The listing builds one solid part. Answer for the finished solid, in the listing's coordinates (mm). Face numbers are marked on the shaded views. A direction names the side the tool comes from. Coordinates: 2 decimals unless noted, no trailing zeros. Loops run counter-clockwise (first coordinate to the right, second up) from the corner with the lowest first, then second, coordinate; pieces in that order, holes last. Notation, with made-up numbers: (53, 79.5) - (82, 79.5) arc R15 ccw to (82, 99.5) - close; hole circle Ø3 at (41, 53.5). An arc over 180 degrees is marked (long way). Return JSON: item names as keys, results as strings. Group by question number.
1. Which of the six approach directions +Z, -Z, +X, -X, +Y, -Y give full straight-line access (tool end or side, diameter ignored) to the marked faces 1 and 2?
2. Section A-A (x = 0) is taken. Write down the section's boundary in (y, z).
3. Find the intervals of material crossed by line 1 along X through (y, z) = (29, 1); line 2 along Y through (x, z) = (65, 4.5); line 3 along Z through (x, y) = (-253.5, 48.5), in increasing order.
4. Section C-C (x = 407) is taken. Write down the section's boundary in (y, z).
5. Section B-B (z = 16.25) is taken. Write down the section's boundary in (x, y).
6. Each of these flat-tipped pins is pushed along its axis until it touches: P1, Ø12, axis at x = 45, z = 12, coming from the +Y side; P2, Ø1.6, axis at x = -244.5, z = 1, coming from the +Y side; P3, Ø6, axis at x = -341.5, y = 37, coming from the +Z side. Where does it stop, or does it pass through?
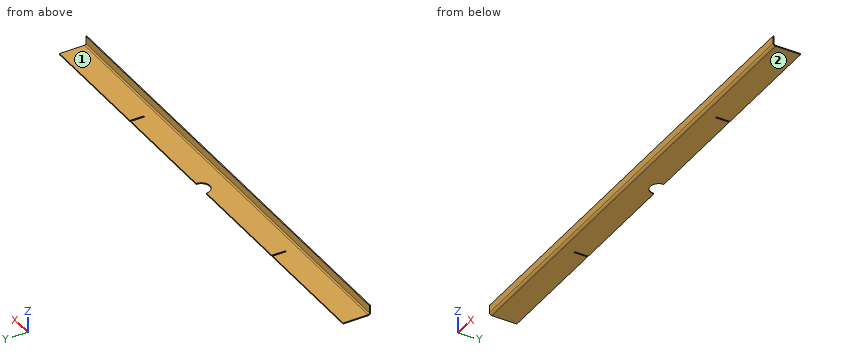
Autodesk Inventor part; units mm, degrees
ref_plane "YZ Plane" through (0, 0, 0) normal (1, 0, 0) x (0, 1, 0)
ref_plane "XZ Plane" through (0, 0, 0) normal (0, 1, 0) x (-1, 0, 0)
ref_plane "XY Plane" through (0, 0, 0) normal (0, 0, 1) x (1, 0, 0)
sketch "Sketch1" plane through (0, 0, 0) normal (0, 0, 1) x (1, 0, 0)
  line L0 (-490, 54) -> (490, 54)
  line L1 (490, 54) -> (490, 0)
  line L2 (490, 0) -> (-490, 0)
  line L3 (-490, 0) -> (-490, 54)
  point P0 (0, 0)
  point P1 (0, 0)
  dimension "d0" = 980
  dimension "d1" = 54
extrude "Plate1" add sketch "Sketch1" along normal blind 2
sketch "Sketch2" plane through (490, -2, 0) normal (0, 1, 0) x (-1, 0, 0)
  line L0 (980, 0) -> (0, 0)
  line L1 (0, 0) -> (0, 20)
  line L2 (0, 20) -> (980, 20)
  line L3 (980, 20) -> (980, 0)
edge flange "Flange1" height 20 angle 90 thickness 2 bend radius 2.75 thickness toward (0, 1, 0) relief round relief width 2 relief depth 1 edges at (0, 0, 2) wall of the first edge with corners at (-490, -2, 0) (490, -2, 0) (490, -2, 20) (-490, -2, 20)
bend "Bend1"
corner "Corner1"
sketch "Sketch5" plane through (0, 0, 0) normal (0, 0, -1) x (-1, 0, 0)
  line L0 (490, 54) -> (-490, 54)
  line L1 (490, -2) -> (-490, -2)
  circle A0 centre (0, 54) radius 17.5
  line L2 (243.4, 54) -> (246.6, 54)
  line L3 (246.6, 54) -> (246.6, 26)
  line L4 (246.6, 26) -> (243.4, 26)
  line L5 (243.4, 26) -> (243.4, 54)
  line L6 (-243.4, 54) -> (-246.6, 54)
  line L7 (-246.6, 54) -> (-246.6, 26)
  line L8 (-246.6, 26) -> (-243.4, 26)
  line L9 (-243.4, 26) -> (-243.4, 54)
  line L10 (0, 54) -> (0, -2) construction
  point P0 (0, 0)
  point P1 (-490, -2)
  point P2 (245, 26)
  point P3 (-245, 26)
  point P4 (246.6, 54)
  point P5 (-17.5, 54)
  point P6 (17.5, 54)
  point P7 (-246.6, 54)
  dimension "d45" = 35
  dimension "d48" = 3.2
  dimension "d49" = 490
  dimension "d51" = 28
  dimension "d52" = 28
extrude "Extrusion1" cut sketch "Sketch5" against normal through all contours L3 L4 L5 L0 | L9 L8 L7 L0 | A0 L0 picked at (-2.238, 47.1497)
sketch "Sketch9" plane through (0, 0, 2) normal (0, 0, 1) x (1, 0, 0)
  line L0 (485.6141, 29.596) -> (485.6141, 17.596) construction
  line L1 (485.6141, 17.596) -> (285.6141, 17.596) construction
  line L2 (285.6141, 17.596) -> (285.6141, 29.596) construction
  line L3 (285.6141, 29.596) -> (485.6141, 29.596) construction
  line L4 (-490, 54) -> (490, 54)
  point P0 (0, 0)
  point P1 (1.05, 68)
  point P2 (490, 54)
  dimension "d40" = 200
  dimension "d41" = 12
mark "Mark2"
equation "\"d2\" = Thickness"
equation "\"d3\" = BendReliefWidth"
equation "\"d4\" = BendReliefDepth"
equation "\"d5\" = MinimumRemnant"
equation "\"d6\" = TransitionRadius"
equation "\"d9\" = BendRadius"
equation "\"d10\" = CornerReliefSize"
equation "\"d11\" = GapSize"
equation "\"d12\" = JacobiRadiusSize"
equation "\"BendReliefWidth\" = Thickness"
equation "\"BendReliefDepth\" = 0.5 * Thickness"
equation "\"CornerReliefSize\" = 4 * Thickness"
equation "\"MinimumRemnant\" = 2 * Thickness"
equation "\"TransitionRadius\" = BendRadius"
equation "\"JacobiRadiusSize\" = BendRadius"
equation "\"GapSize\" = Thickness"
properties part number "MSC 329 STRINGER BOARD  ###" material "Stainless Steel"
The answers:
{
 "1": {"face 1": "+Z, +X, -X, +Y", "face 2": "-Z, +X, -X, +Y, -Y"},
 "2": {"outline": "(-2, 4.75) arc R4.75 ccw to (2.75, 0) - (36.5, 0) - (36.5, 2) - (2.75, 2) arc R2.75 cw to (0, 4.75) - (0, 20) - (-2, 20) - close"},
 "3": {"line 1": "x = -490 to -246.6, -243.4 to 243.4, 246.6 to 490", "line 2": "y = -1.99 to 0.01", "line 3": "z = 0 to 2"},
 "4": {"outline": "(-2, 4.75) arc R4.75 ccw to (2.75, 0) - (54, 0) - (54, 2) - (2.75, 2) arc R2.75 cw to (0, 4.75) - (0, 20) - (-2, 20) - close"},
 "5": {"outline": "(-490, -2) - (490, -2) - (490, 0) - (-490, 0) - close"},
 "6": {"P1": "stops at y = 0", "P2": "stops at y = 26", "P3": "stops at z = 2"}
}
